Input: part model. Units: mm. Frame: model coordinates. Face numbers are marked on the shaded views. A direction names the side the tool comes from. Coordinates: 2 decimals unless noted, no trailing zeros. Order: outer loops, then holes, each group sorted by start corner. A loop starts at its lowest first (then second) coordinate and runs counter-clockwise, first axis right, second up. Notation, with made-up numbers: (8, 77.5) -> (35, 77.5) arc R22 ccw to (35, 89.5) -> close; hole circle Ø1 at (58.5, -23). An arc over 180 degrees is marked (long way). Answer as CSV lines item,"result".
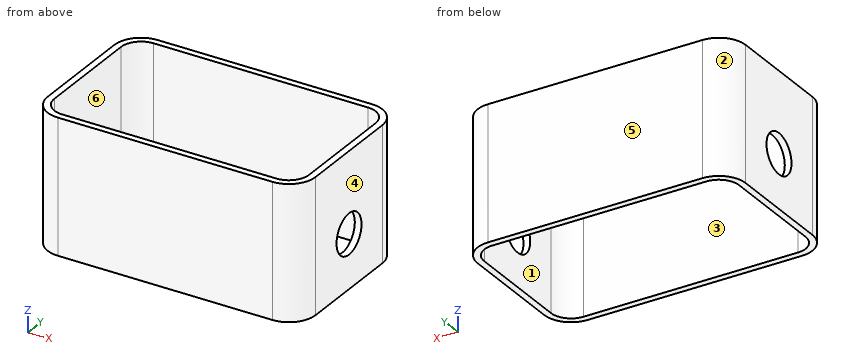
from build123d import *

# Parameters (mm, degrees)
F0_W     = 100
F0_H     = 60
F1_DEPTH = 50
F2_R     = 10
F3_T     = -2.5
F4_R     = 7.5
F5_DEPTH = 119.1


with BuildPart() as f1:
    # F0 (on Top) → F1 (new body)
    with BuildSketch(Plane.XY):
        Rectangle(F0_W, F0_H)
    extrude(amount=F1_DEPTH)

    # F2
    f2_edges = [f1.edges().sort_by_distance(p)[0] for p in [
        (50, -30, 25),
        (50, 30, 25),
        (-50, 30, 25),
        (-50, -30, 25),
    ]]
    fillet(f2_edges, radius=F2_R)

    # F3
    f3_openings = [f1.faces().sort_by_distance(p)[0] for p in [
        (0, 0, 50),
        (0, 0, 0),
    ]]
    offset(amount=F3_T, openings=f3_openings)

    # F4 (on face) → F5 (cut)
    with BuildSketch(Plane(origin=(-50, 0, 0), x_dir=(0, -1, 0), z_dir=(-1, 0, 0))):
        with Locations((0, 20)):
            Circle(F4_R)
    extrude(amount=-F5_DEPTH, mode=Mode.SUBTRACT)


solid = f1.part
1. Cut plane A-A (z = 20). Return the cut outline in (x, y).
Findings:
outline,"(-50, -20) arc R10 ccw to (-40, -30) -> (40, -30) arc R10 ccw to (50, -20) -> (50, -7.5) -> (47.5, -7.5) -> (47.5, -20) arc R7.5 cw to (40, -27.5) -> (-40, -27.5) arc R7.5 cw to (-47.5, -20) -> (-47.5, -7.5) -> (-50, -7.5) -> close; (-50, 7.5) -> (-47.5, 7.5) -> (-47.5, 20) arc R7.5 cw to (-40, 27.5) -> (40, 27.5) arc R7.5 cw to (47.5, 20) -> (47.5, 7.5) -> (50, 7.5) -> (50, 20) arc R10 ccw to (40, 30) -> (-40, 30) arc R10 ccw to (-50, 20) -> close"
2. Reachability of the marked faces 5 and 6 from +Z, -Z, +X, -X, +Y, -Y: full face, straight path, thin tool, end or side. Return the list, or none.
Findings:
face 5,"+Z, -Z, +X, -X, +Y"
face 6,"+Z, -Z"
3. Cut plane D-D (y = 0). Return the cut outline in (x, z).
Findings:
outline,"(-50, 0) -> (-47.5, 0) -> (-47.5, 12.5) -> (-50, 12.5) -> close; (-50, 27.5) -> (-47.5, 27.5) -> (-47.5, 50) -> (-50, 50) -> close; (47.5, 0) -> (50, 0) -> (50, 12.5) -> (47.5, 12.5) -> close; (47.5, 27.5) -> (50, 27.5) -> (50, 50) -> (47.5, 50) -> close"
4. Mould query, pull axis X, two halves, no side actions, for the marked faces 1, 2, 3 and 4. Classes: released by +X, released by -X, zero draft, split by the parting line, or undercut.
Findings:
face 1,"undercut"
face 2,"released by -X"
face 3,"undercut"
face 4,"released by +X"
5. Ray query, line 1 along Z through (x, y) = (49.05, 0); line 2 along Y through (x, z) = (-19, 42); line 3 along X through (y, z) = (-12.5, 3.5). Return the intervals inside material, ascending.
Findings:
line 1,"z = 0 to 12.5, 27.5 to 50"
line 2,"y = -30 to -27.5, 27.5 to 30"
line 3,"x = -50 to -47.5, 47.5 to 50"
6. Cut plane B-B (y = -18.5). Return the cut outline in (x, z).
Findings:
outline,"(-50, 0) -> (-47.5, 0) -> (-47.5, 50) -> (-50, 50) -> close; (47.5, 0) -> (50, 0) -> (50, 50) -> (47.5, 50) -> close"
7. Cut plane C-C (x = -38.5). Return the cut outline in (y, z), plus the area to 3 significant figures.
Findings:
outline,"(-30, 0) -> (-27.5, 0) -> (-27.5, 50) -> (-30, 50) -> close; (27.5, 0) -> (30, 0) -> (30, 50) -> (27.5, 50) -> close"
area,"250 mm2"
8. Contact query for a flat-ended pin moving along its axis: pin 1 (24 mm diameter, centred on y = 0, z = 20, fed in from +X). Output: stop coordinate, or through.
Findings:
pin 1,"stops at x = 50"
